from build123d import *

# Parameters (mm, degrees)
ESQUISSE1_W             = 160
ESQUISSE1_H             = 440
ESQUISSE1_R             = 2.2
ESQUISSE1_W_2           = 110
ESQUISSE1_H_2           = 160
BOSS_EXTRU_1_DEPTH      = 4
ESQUISSE2_R             = 2.2
ESQUISSE2_W             = 160
ESQUISSE2_H             = 120
ENL_V_MAT_EXTRU_1_DEPTH = 5


with BuildPart() as part:
    # Esquisse1 → Boss.-Extru.1 (new body)
    with BuildSketch(Plane.XY):
        Rectangle(ESQUISSE1_W, ESQUISSE1_H)
        with Locations((70, 0)):
            Circle(ESQUISSE1_R, mode=Mode.SUBTRACT)
        with Locations((70, 210)):
            Circle(ESQUISSE1_R, mode=Mode.SUBTRACT)
        with Locations((70, -210)):
            Circle(ESQUISSE1_R, mode=Mode.SUBTRACT)
        with Locations((-70, 210)):
            Circle(ESQUISSE1_R, mode=Mode.SUBTRACT)
        with Locations((-70, 0)):
            Circle(ESQUISSE1_R, mode=Mode.SUBTRACT)
        with Locations((-70, -210)):
            Circle(ESQUISSE1_R, mode=Mode.SUBTRACT)
        with Locations((0, 110)):
            Rectangle(ESQUISSE1_W_2, ESQUISSE1_H_2, mode=Mode.SUBTRACT)
    extrude(amount=BOSS_EXTRU_1_DEPTH)

    # Esquisse2 → Enlèv. mat.-Extru.1 (cut, through all)
    with BuildSketch(Plane.XY.offset(4)):
        with Locations((-70, -90)):
            Circle(ESQUISSE2_R)
        with Locations((70, -90)):
            Circle(ESQUISSE2_R)
        with Locations((0, -160)):
            Rectangle(ESQUISSE2_W, ESQUISSE2_H)
    extrude(amount=-ENL_V_MAT_EXTRU_1_DEPTH, mode=Mode.SUBTRACT)


solid = part.part
Design review of the part built by this model. Coordinates are the model's own, in mm. Give positions to 0.01 mm unless a question says otherwise; leave off trailing zeros. Write each loop counter-clockwise with the first axis right and the second up, starting at its lowest first coordinate (ties: lowest second). Pieces come first, ordered by that corner, then holes. Notation, with made-up numbers: M 11.5,36 L 23.5,36 A10 cw 23.5,49 Z; hole C -0.5,79.5 d11. An arc over 180 degrees is marked long. Answer as a JSON object with one key per item and string values. Group by question number.
1) We need section B-B (x = -44.5). Give the boundary of the cut face in (y, z).
2) We need section A-A (y = 59). Give the boundary of the cut face in (x, z), and give its area (3 significant figures).
3) We need section C-C (z = 2.1). Give the boundary of the cut face in (x, y), and give its area (3 significant figures).
4) Clearance check with a flat-ended pin moving along its axis: pin 1 Ø5 at (x, y) = (70, -90) entering from +Z. State where the tip first meets the part, or that it passes through.
5) For line 1 along Y through (x, z) = (70, 0.75); line 2 along X through (y, z) = (210, 1.4); line 3 along Y through (x, z) = (6, 1.7), list the stretches that pass through material, from the lowest coordinate up.
Answer key:
{
 "1": {"outline": "M -100,0 L 30,0 L 30,4 L -100,4 Z; M 190,0 L 220,0 L 220,4 L 190,4 Z"},
 "2": {"outline": "M -80,0 L -55,0 L -55,4 L -80,4 Z; M 55,0 L 80,0 L 80,4 L 55,4 Z", "area": "200 mm²"},
 "3": {"outline": "M -80,-100 L 80,-100 L 80,220 L -80,220 Z; hole C -70,-90 d4.4; hole C -70,0 d4.4; hole C -70,210 d4.4; hole M -55,30 L 55,30 L 55,190 L -55,190 Z; hole C 70,-90 d4.4; hole C 70,0 d4.4; hole C 70,210 d4.4", "area": "33,500 mm²"},
 "4": {"pin 1": "stops at z = 4"},
 "5": {"line 1": "y = -100 to -92.2, -87.8 to -2.2, 2.2 to 207.8, 212.2 to 220", "line 2": "x = -80 to -72.2, -67.8 to 67.8, 72.2 to 80", "line 3": "y = -100 to 30, 190 to 220"}
}
